Read the model definition and answer for the solid it produces. Units are mm, in the model's axes. Face numbers are marked on the shaded views. A direction names the side the tool comes from. Coordinates: 2 decimals unless noted, no trailing zeros. Write each loop counter-clockwise with the first axis right and the second up, starting at its lowest first coordinate (ties: lowest second). Pieces come first, ordered by that corner, then holes. Notation, with made-up numbers: M -10,2.25 L 43,2.25 A35 ccw 43,36.25 Z; hole C 86,53 d11. An arc over 180 degrees is marked long. Use a Markdown table: item, result. Add a question column.
from build123d import *

# Parameters (mm, degrees)
SKETCH_1_W          = 51
SKETCH_1_H          = 50
EXTRUDE_1_DEPTH     = 25
SKETCH_2_R          = 10
CUT_EXTRUDE_1_DEPTH = 26
SKETCH_3_W          = 45
SKETCH_3_H          = 44
CUT_EXTRUDE_2_DEPTH = 21
SKETCH_4_W          = 81
SKETCH_4_H          = 25
SKETCH_4_R          = 5
EXTRUDE_2_DEPTH     = 3


with BuildPart() as part:
    # 草圖1 → 填料-伸長1 (new body)
    with BuildSketch(Plane(origin=(0, 0, 0), x_dir=(1, 0, 0), z_dir=(0, 1, 0))):
        Rectangle(SKETCH_1_W, SKETCH_1_H)
    extrude(amount=EXTRUDE_1_DEPTH)

    # 草圖2 → 除料-伸長1 (cut, through all)
    with BuildSketch(Plane(origin=(0, 25, 0), x_dir=(1, 0, 0), z_dir=(0, 1, 0))):
        Circle(SKETCH_2_R)
    extrude(amount=-CUT_EXTRUDE_1_DEPTH, mode=Mode.SUBTRACT)

    # 草圖3 → 除料-伸長2 (cut)
    with BuildSketch(Plane(origin=(0, 25, 0), x_dir=(1, 0, 0), z_dir=(0, 1, 0))):
        Rectangle(SKETCH_3_W, SKETCH_3_H)
    extrude(amount=-CUT_EXTRUDE_2_DEPTH, mode=Mode.SUBTRACT)

    # 草圖4 → 填料-伸長2 (add)
    with BuildSketch(Plane(origin=(0, 0, 22), x_dir=(-1, 0, 0), z_dir=(0, 0, -1))):
        with Locations((0, 12.5)):
            Rectangle(SKETCH_4_W, SKETCH_4_H)
        with Locations((-33, 12.5)):
            Circle(SKETCH_4_R, mode=Mode.SUBTRACT)
        with Locations((33, 12.5)):
            Circle(SKETCH_4_R, mode=Mode.SUBTRACT)
    extrude(amount=-EXTRUDE_2_DEPTH)


solid = part.part
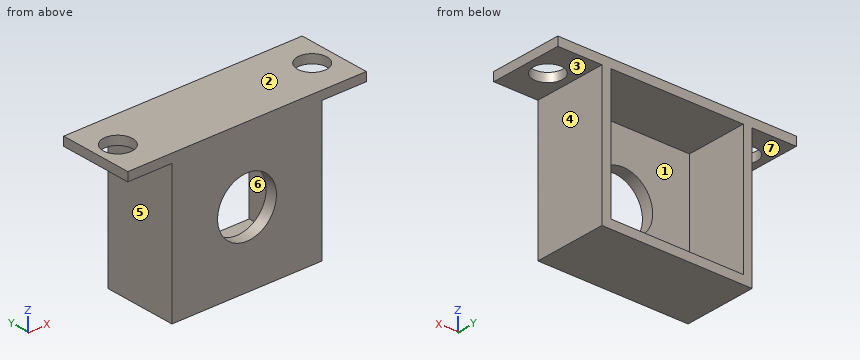
Item 1: Find section D-D on y = 2.75. Give the vertices of the cut face in (x, z), then the cut area to 3 significant figures.
Item 2: Find section B-B on x = 33. Give the vertices of the cut face in (y, z), then the cut area to 3 significant figures.
Item 3: Determine the mould class of the marked faces 4, 5, 6 and 7 for opening direction X: pulls with the +X half, pulls with the -X half, needs draft (parallel to the pull), parting line crosses it, or undercut.
Item 4: Find section A-A on y = 12.5. Give the vertices of the cut face in (x, z), then the cut area to 3 significant figures.
Item 5: Each of these flat-tipped pins is pushed along its axis until it touches: pin 1 (8 mm diameter, centred on x = 14.5, z = 8, fed in from +Y); pin 2 (7.5 mm diameter, centred on y = 7.5, z = -7.5, fed in from +X); pin 3 (7.5 mm diameter, centred on x = 36.5, y = 13, fed in from -Z); pin 4 (4 mm diameter, centred on x = -26, z = -18, fed in from +Y). Where does it stop, or does it pass through?
Item 6: Consider probe 1 along Z at (x, y) = (-3, 21.25); probe 2 along Z at (x, y) = (0, 1.15); probe 3 along Y at (x, z) = (33, 23.8). Determine where each line is inside the solid, lowest interval first.
Item 7: Find section C-C on z = 0. Give the vertices of the cut face in (x, y), then the cut area to 3 significant figures.
Item 8: For the marked faces 1, 2 and 3, determine the directions among +Z, -Z, +X, -X, +Y, -Y from which every point of the face is accessible in a straight line to the end or side of a thin tool.
Geometry says:
| question | item | result |
|---|---|---|
| 1 | outline | M -40.5,22 L -25.5,22 L -25.5,-25 L 25.5,-25 L 25.5,22 L 40.5,22 L 40.5,25 L -40.5,25 Z; hole C 0,0 d20 |
| 1 | area | 2,330 mm2 |
| 2 | outline | M 0,22 L 7.5,22 L 7.5,25 L 0,25 Z; M 17.5,22 L 25,22 L 25,25 L 17.5,25 Z |
| 2 | area | 45.0 mm2 |
| 3 | face 4 | pulls with the +X half |
| 3 | face 5 | pulls with the -X half |
| 3 | face 6 | undercut |
| 3 | face 7 | needs draft |
| 4 | outline | M -40.5,22 L -38,22 L -38,25 L -40.5,25 Z; M -28,22 L -25.5,22 L -25.5,-25 L 25.5,-25 L 25.5,22 L 28,22 L 28,25 L -28,25 Z; M 38,22 L 40.5,22 L 40.5,25 L 38,25 Z; hole M -22.5,-22 L 22.5,-22 L 22.5,22 L -22.5,22 Z |
| 4 | area | 600 mm2 |
| 5 | pin 1 | stops at y = 4 |
| 5 | pin 2 | stops at x = 25.5 |
| 5 | pin 3 | stops at z = 22 |
| 5 | pin 4 | stops at y = 25 |
| 6 | probe 1 | z = -25 to -22, 22 to 25 |
| 6 | probe 2 | z = -25 to -10, 10 to 25 |
| 6 | probe 3 | y = 0 to 7.5, 17.5 to 25 |
| 7 | outline | M -25.5,0 L -10,0 L -10,4 L -22.5,4 L -22.5,25 L -25.5,25 Z; M 10,0 L 25.5,0 L 25.5,25 L 22.5,25 L 22.5,4 L 10,4 Z |
| 7 | area | 250 mm2 |
| 8 | face 1 | +Y |
| 8 | face 2 | +Z, +X, -X, +Y, -Y |
| 8 | face 3 | -Z, +X, +Y, -Y |
